from build123d import *

# Parameters (mm, degrees)
SKETCH1_W           = 110
SKETCH1_H           = 70
SKETCH1_R           = 1.75
BOSS_EXTRUDE1_DEPTH = 2
SKETCH2_W           = 7
SKETCH2_H           = 19.5
CUT_EXTRUDE1_DEPTH  = 66.222695436
FILLET1_R           = 3
SKETCH3_R           = 1.5
CUT_EXTRUDE2_DEPTH  = 66.222695436


with BuildPart() as part:
    # Sketch1 → Boss-Extrude1 (new body)
    with BuildSketch(Plane(origin=(0, 0, 0), x_dir=(1, 0, 0), z_dir=(0, 1, 0))):
        Rectangle(SKETCH1_W, SKETCH1_H)
        with Locations(Location((-50, 30, 0), (0, 0, 270))):
            Circle(SKETCH1_R, mode=Mode.SUBTRACT)
        with Locations(Location((-50, -30, 0), (0, 0, 270))):
            Circle(SKETCH1_R, mode=Mode.SUBTRACT)
        with Locations(Location((50, -30, 0), (0, 0, 270))):
            Circle(SKETCH1_R, mode=Mode.SUBTRACT)
        with Locations(Location((50, 30, 0), (0, 0, 270))):
            Circle(SKETCH1_R, mode=Mode.SUBTRACT)
        Polygon((39.984778377, 28.64285469), (-45.603033207, 28.64285469), (-45.603033207, 8.299784998), (-44.51, 8.299784998), (-44.51, -8.200215002), (-45.603033207, -8.200215002), (-45.603033207, -28.591287888), (39.984778377, -28.591287888), (39.984778377, -8.200215002), (38.89, -8.200215002), (38.89, 8.299784998), (39.984778377, 8.299784998), align=None, mode=Mode.SUBTRACT)
    extrude(amount=BOSS_EXTRUDE1_DEPTH)

    # Sketch2 → Cut-Extrude1 (cut, through all)
    with BuildSketch(Plane(origin=(0, 2, 0), x_dir=(1, 0, 0), z_dir=(0, 1, 0))):
        with Locations((48, 0)):
            Rectangle(SKETCH2_W, SKETCH2_H)
    extrude(amount=-CUT_EXTRUDE1_DEPTH, mode=Mode.SUBTRACT)

    # Fillet1
    fillet1_edges = [part.edges().sort_by_distance(p)[0] for p in [
        (-55, 1, -35),
        (55, 1, -35),
        (55, 1, 35),
        (-55, 1, 35),
    ]]
    fillet(fillet1_edges, radius=FILLET1_R)

    # Sketch3 → Cut-Extrude2 (cut, through all)
    with BuildSketch(Plane.XZ):
        with Locations(Location((50, 22, 0), (0, 0, 270))):
            Circle(SKETCH3_R)
        with Locations(Location((-50, -22, 0), (0, 0, 270))):
            Circle(SKETCH3_R)
    extrude(amount=-CUT_EXTRUDE2_DEPTH, mode=Mode.SUBTRACT)


solid = part.part
Geometry check sheet. Reference: the model listing, model coordinates, mm. A direction names the side the tool comes from. Give positions to 0.01 mm unless a question says otherwise; leave off trailing zeros. Loops run counter-clockwise (first coordinate to the right, second up) from the corner with the lowest first, then second, coordinate; pieces in that order, holes last. Notation, with made-up numbers: M 14,4 L 44,4 A37 ccw 44,40 Z; hole C -12.75,2.25 d5. An arc over 180 degrees is marked long. Answer as a JSON object with one key per item and string values. Group by question number.
Item 1: Sectioned sample at B-B on z = -22. Record the boundary of the cut face in (x, y), plus the area to 3 significant figures.
Item 2: Access from +Z, -Z, +X, -X, +Y, -Y to the whole of each face (thin tool, end or side, straight path). Record for faces 1 (the flat face through (38.89, 1, 0)), 2 (the flat face through (-1, 1, -35)).
Item 3: Material ranges on L1, parallel to X at y = 1.2, z = 22; L2, parallel to X at y = 0.65, z = -22; L3, parallel to Z at x = -4, y = 0.6, recorded low to high.
Item 4: Sectioned sample at A-A on x = -50. Record the boundary of the cut face in (y, z), plus the area to 3 significant figures.
Item 5: Sectioned sample at C-C on x = -11.5. Record the boundary of the cut face in (y, z), plus the area to 3 significant figures.
Item 6: Gauge pin test, flat end, axial feed: pin 1 (5.5 mm diameter, centred on x = -50, z = -30, fed in from -Y). Record the tip position at first contact, or that the pin passes through.
Item 7: Mould release check, pull along X, two halves, no side actions. Record for faces 3 (the flat face through (55, 1, 0)), 4 (the cylindrical face through (-51.06, 0.99, -31.39)), 5 (the flat face through (4, 2, -29)): pulls with the +X half, pulls with the -X half, needs draft (parallel to the pull), parting line crosses it, or undercut.
Item 8: Sectioned sample at D-D on x = 50. Record the boundary of the cut face in (y, z).
Findings below:
{
 "1": {"outline": "M -55,0 L -51.5,0 L -51.5,2 L -55,2 Z; M -48.5,0 L -45.6,0 L -45.6,2 L -48.5,2 Z; M 39.98,0 L 55,0 L 55,2 L 39.98,2 Z", "area": "42.8 mm2"},
 "2": {"face 1": "+Y, -Y", "face 2": "-Z, +X, -X, +Y, -Y"},
 "3": {"L1": "-55 to -45.6, 39.98 to 48.5, 51.5 to 55", "L2": "-55 to -51.5, -48.5 to -45.6, 39.98 to 55", "L3": "-35 to -28.64, 28.59 to 35"},
 "4": {"outline": "M 0,-35 L 2,-35 L 2,-31.75 L 0,-31.75 Z; M 0,-28.25 L 2,-28.25 L 2,-23.5 L 0,-23.5 Z; M 0,-20.5 L 2,-20.5 L 2,28.25 L 0,28.25 Z; M 0,31.75 L 2,31.75 L 2,35 L 0,35 Z", "area": "120 mm2"},
 "5": {"outline": "M 0,-35 L 2,-35 L 2,-28.64 L 0,-28.64 Z; M 0,28.59 L 2,28.59 L 2,35 L 0,35 Z", "area": "25.5 mm2"},
 "6": {"pin 1": "y = 0"},
 "7": {"face 3": "pulls with the +X half", "face 4": "undercut", "face 5": "needs draft"},
 "8": {"outline": "M 0,-35 L 2,-35 L 2,-31.75 L 0,-31.75 Z; M 0,-28.25 L 2,-28.25 L 2,-9.75 L 0,-9.75 Z; M 0,9.75 L 2,9.75 L 2,20.5 L 0,20.5 Z; M 0,23.5 L 2,23.5 L 2,28.25 L 0,28.25 Z; M 0,31.75 L 2,31.75 L 2,35 L 0,35 Z"}
}
